from build123d import *

# Parameters (mm, degrees)
CONTROL_BATTERY_CLAMP_START = 94
SKETCH_1_W                  = 10
SKETCH_1_H                  = 92
CONTROL_BATTERY_CLAMP_DEPTH = 4
CLAMP_TWO_M3_START          = 99
SKETCH_2_R                  = 1.7
CLAMP_TWO_M3_DEPTH          = 6


with BuildPart() as part:
    # 草图1 → Control_battery_clamp (new body)
    with BuildSketch(Plane.XY.offset(CONTROL_BATTERY_CLAMP_START)):
        with Locations((80, 0)):
            Rectangle(SKETCH_1_W, SKETCH_1_H)
    extrude(amount=CONTROL_BATTERY_CLAMP_DEPTH)

    # 草图2 → Clamp_two_M3 (cut)
    with BuildSketch(Plane.XY.offset(CLAMP_TWO_M3_START)):
        with Locations(Location((80, -41, 0), (0, 0, 180))):
            Circle(SKETCH_2_R)
        with Locations(Location((80, 41, 0), (0, 0, 180))):
            Circle(SKETCH_2_R)
    extrude(amount=-CLAMP_TWO_M3_DEPTH, mode=Mode.SUBTRACT)


solid = part.part
Geometry check sheet. Reference: the model listing, model coordinates, mm. Give positions to 0.01 mm unless a question says otherwise; leave off trailing zeros. Loops run counter-clockwise (first coordinate to the right, second up) from the corner with the lowest first, then second, coordinate; pieces in that order, holes last. Notation, with made-up numbers: M -36,-25.5 L -16,-25.5 A14 ccw -16,-15.5 Z; hole C 74,47.5 d5. An arc over 180 degrees is marked long. Answer as a JSON object with one key per item and string values. Group by question number.
Item 1: Sectioned sample at A-A on y = -41. Record the boundary of the cut face in (x, z).
Item 2: Sectioned sample at B-B on x = 80. Record the boundary of the cut face in (y, z), plus the area to 3 significant figures.
Item 3: Sectioned sample at C-C on z = 96.75. Record the boundary of the cut face in (x, y), plus the area to 3 significant figures.
Item 4: Material ranges on L1, parallel to Y at x = 80, z = 95.8; L2, parallel to Y at x = 78.75, z = 95.2; L3, parallel to X at y = -41, z = 96.15, recorded low to high.
Item 5: Mould release check, pull along Y, two halves, no side actions. Record for faces 1 (the cylindrical face through (81.7, -41.07, 96.03)), 2 (the flat face through (80, 46, 96)), 3 (the cylindrical face through (81.7, 40.93, 96.03)), 4 (the flat face through (85, -1, 96)): pulls with the +Y half, pulls with the -Y half, needs draft (parallel to the pull), parting line crosses it, or undercut.
Findings below:
{
 "1": {"outline": "M 75,94 L 78.3,94 L 78.3,98 L 75,98 Z; M 81.7,94 L 85,94 L 85,98 L 81.7,98 Z"},
 "2": {"outline": "M -46,94 L -42.7,94 L -42.7,98 L -46,98 Z; M -39.3,94 L 39.3,94 L 39.3,98 L -39.3,98 Z; M 42.7,94 L 46,94 L 46,98 L 42.7,98 Z", "area": "341 mm2"},
 "3": {"outline": "M 75,-46 L 85,-46 L 85,46 L 75,46 Z; hole C 80,-41 d3.4; hole C 80,41 d3.4", "area": "902 mm2"},
 "4": {"L1": "-46 to -42.7, -39.3 to 39.3, 42.7 to 46", "L2": "-46 to -42.15, -39.85 to 39.85, 42.15 to 46", "L3": "75 to 78.3, 81.7 to 85"},
 "5": {"face 1": "undercut", "face 2": "pulls with the +Y half", "face 3": "undercut", "face 4": "needs draft"}
}
